Part model, mm, in its own coordinate system. A direction names the side the tool comes from. Round coordinates to 2 decimals unless told otherwise and drop trailing zeros. Order: outer loops, then holes, each group sorted by start corner. A loop starts at its lowest first (then second) coordinate and runs counter-clockwise, first axis right, second up. Notation, with made-up numbers: (10, 62.25) -> (23, 62.25) arc R17 cw to (23, 91.25) -> close; hole circle Ø9 at (-39.75, 44). An arc over 180 degrees is marked (long way). Use CSV: the item, a comma, the result in double quotes.
```python
from build123d import *

# Parameters (mm, degrees)
F1_DEPTH  = 76.2
F2_R      = 16.759679
F3_DEPTH  = 50.801
F4_R      = 10.122636
F5_DEPTH  = 76.201
F6_R      = 28.758391
F7_DEPTH  = 114.301
F8_R      = 5.08
F10_W     = 15.888512
F10_H     = 3.972126
F11_DEPTH = 25.4
F13_DEPTH = 2.54


with BuildPart() as f1:
    # F0 (on Front) → F1 (new body)
    with BuildSketch(Plane.XZ):
        Polygon((-44.173401, -27.656091), (-44.173401, -53.056091), (32.026599, -53.056091), (32.026599, -27.656091), (6.626599, -27.656091), (6.626599, 35.843909), (32.026599, 35.843909), (32.026599, 61.243909), (-44.173401, 61.243909), (-44.173401, 35.843909), (-18.773401, 35.843909), (-18.773401, -27.656091), align=None)
    extrude(amount=F1_DEPTH)

    # F2 (on face) → F3 (cut, through all)
    with BuildSketch(Plane.YZ.offset(6.626599)):
        with Locations((-43.022785, 3.559439)):
            Circle(F2_R)
    extrude(amount=-F3_DEPTH, mode=Mode.SUBTRACT)

    # F4 (on face) → F5 (cut, through all)
    with BuildSketch(Plane.XZ.offset(76.2)):
        with Locations((-5.116025, 4.186992)):
            Circle(F4_R)
    extrude(amount=-F5_DEPTH, mode=Mode.SUBTRACT)

    # F6 (on face) → F7 (cut, through all)
    with BuildSketch(Plane(origin=(0, 0, -53.056091), x_dir=(1, 0, 0), z_dir=(0, 0, -1))):
        with Locations((-5.880812, 38.534798)):
            Circle(F6_R)
    extrude(amount=-F7_DEPTH, mode=Mode.SUBTRACT)

    # F8
    f8_edges = [f1.edges().sort_by_distance(p)[0] for p in [
        (-6.073401, -76.2, 61.243909),
        (32.026599, -38.1, 61.243909),
        (32.026599, -76.2, 48.543909),
        (-6.073401, 0, 61.243909),
        (32.026599, 0, 48.543909),
        (-44.173401, 0, 48.543909),
        (-44.173401, -38.1, 61.243909),
    ]]
    fillet(f8_edges, radius=F8_R)

    # F10 (on face) → F11 (join)
    with BuildSketch(Plane.XY.offset(61.243909)):
        with Locations((-29.480584, -11.146277)):
            Rectangle(F10_W, F10_H)
    extrude(amount=F11_DEPTH)

    # F12 (on face) → F13 (cut)
    with BuildSketch(Plane(origin=(0, -9.160214, 0), x_dir=(-1, 0, 0), z_dir=(0, 1, 0))):
        Polygon((33.161537, 67.962763), (36.611519, 74.066582), (33.050448, 80.106264), (26.039395, 80.042126), (22.589412, 73.938308), (26.150483, 67.898626), align=None)
    extrude(amount=-F13_DEPTH, mode=Mode.SUBTRACT)


solid = f1.part
```
(1) Cut at D-D, the plane y = -69.5. Give the cut face in (x, z), then the cut area to 3 significant figures.
Reply:
outline,"(-44.17, -53.06) -> (32.03, -53.06) -> (32.03, -27.66) -> (6.63, -27.66) -> (6.63, 35.84) -> (32.03, 35.84) -> (32.03, 56.16) arc R5.08 ccw to (26.95, 61.24) -> (-39.09, 61.24) arc R5.08 ccw to (-44.17, 56.16) -> (-44.17, 35.84) -> (-18.77, 35.84) -> (-18.77, -27.66) -> (-44.17, -27.66) -> close; hole circle Ø20.25 at (-5.12, 4.19)"
area,"5,150 mm2"
(2) Drop flat-ended pins along their axis: P1, Ø10, axis at y = -62, z = 20.5, coming from the -X side; P2, Ø17.5, axis at x = -32.5, z = 73.5, coming from the +Y side; P3, Ø12, axis at x = 23.5, y = -18.5, coming from the +Z side; P4, Ø12.5, axis at x = 17.5, y = -47, coming from the -Z side. Give the stop position or say it passes through.
Reply:
P1,"x = -18.77"
P2,"y = -9.16"
P3,"z = 61.24"
P4,"z = -53.06"
(3) Probe probe 1 along Y at (x, z) = (5, -18); probe 2 along Z at (x, y) = (-32, -22.5); probe 3 along Z at (x, y) = (-34, -4). List the from-to ranges inside material, lowest first. Write a range as [from, to].
Reply:
probe 1,"[-76.2, -65.16], [-11.91, 0]"
probe 2,"[-53.06, -27.66], [35.84, 61.24]"
probe 3,"[-53.06, -27.66], [35.84, 61.13]"
(4) Cut at A-A, the plane z = -13.5. Give the cut face in (x, y).
Reply:
outline,"(-18.77, -76.2) -> (6.63, -76.2) -> (6.63, -64.43) arc R28.76 cw to (-18.77, -64.24) -> close; (-18.77, -12.83) arc R28.76 cw to (6.63, -12.64) -> (6.63, 0) -> (-18.77, 0) -> close"
(5) Cut at C-C, the plane x = -5. Give the cut face in (y, z).
Reply:
outline,"(-76.2, -53.06) -> (-67.28, -53.06) -> (-67.28, -5.93) -> (-76.2, -5.93) -> close; (-76.2, 14.31) -> (-67.28, 14.31) -> (-67.28, 61.24) -> (-71.12, 61.24) arc R5.08 ccw to (-76.2, 56.16) -> close; (-9.79, -53.06) -> (0, -53.06) -> (0, -5.93) -> (-9.79, -5.93) -> close; (-9.79, 14.31) -> (0, 14.31) -> (0, 56.16) arc R5.08 ccw to (-5.08, 61.24) -> (-9.79, 61.24) -> close"
(6) Pull direction X, two halves, no side cores. Call faces 1 (the face through (-18.773, -70, 5)), 2 (the face through (-30, -11.7, 74)), 3 (the face through (-30, -11, 86.644)): released by +X, released by -X, zero draft, split by the parting line, or undercut.
Reply:
face 1,"released by -X"
face 2,"undercut"
face 3,"zero draft"
(7) Cut at B-B, the plane y = -20.5. Give the cut face in (x, z), then the cut area to 3 significant figures.
Reply:
outline,"(-44.17, -53.06) -> (-28.28, -53.06) -> (-28.28, -27.66) -> (-44.17, -27.66) -> close; (-44.17, 35.84) -> (-28.28, 35.84) -> (-28.28, 61.24) -> (-39.09, 61.24) arc R5.08 ccw to (-44.17, 56.16) -> close; (16.52, -53.06) -> (32.03, -53.06) -> (32.03, -27.66) -> (16.52, -27.66) -> close; (16.52, 35.84) -> (32.03, 35.84) -> (32.03, 56.16) arc R5.08 ccw to (26.95, 61.24) -> (16.52, 61.24) -> close"
area,"1,580 mm2"
(8) Which spindle directions (+Z, -Z, +X, -X, +Y, -Y) get a long thin tool onto all of the face, cutting with end or side? Do faces 4 (the face through (-34.86, -10.41, 70.97)), 5 (the face through (6.627, -70, 4)), 6 (the face through (32.027, -38, 46)), 7 (the face through (30.5, -1.45, 46.15)), 8 (the face through (-21.536, -11, 74)). Say none if no direction does.
Reply:
face 4,"+Y"
face 5,"+X, +Y, -Y"
face 6,"+Z, -Z, +X, +Y, -Y"
face 7,"+Z, +X, +Y"
face 8,"+Z, +X, +Y, -Y"
